Read the model definition and answer for the solid it produces. Units are mm, in the model's axes. A direction names the side the tool comes from. Coordinates: 2 decimals unless noted, no trailing zeros. Loops run counter-clockwise (first coordinate to the right, second up) from the corner with the lowest first, then second, coordinate; pieces in that order, holes last. Notation, with made-up numbers: (-36, 12) - (4, 12) arc R15 cw to (4, 22) - close; hole circle Ø9 at (78, 36.5). An arc over 180 degrees is marked (long way). Use one line per item in the form item = value.
from build123d import *

# Parameters (mm, degrees)
SKETCH1_W                    = 50.8
SKETCH1_H                    = 38.1
BOSS_EXTRUDE1_DEPTH          = 15.875
F_1_4_20_TAPPED_HOLE1_D      = 5.1054
CUT_EXTRUDE1_DEPTH           = 36.497579143
CUT_EXTRUDE1_DEPTH_BACK      = 36.497579143
SKETCH5_W                    = 73.284203365
SKETCH5_H                    = 114.763304797
CUT_EXTRUDE3_DEPTH           = 36.497579143
CUT_EXTRUDE3_DRAFT           = 45
CUT_EXTRUDE3_PROFILE_2_DEPTH = 36.497579143
CUT_EXTRUDE3_PROFILE_2_DRAFT = 45
CUT_EXTRUDE5_DEPTH           = 34.299680929
CUT_EXTRUDE5_DEPTH_BACK      = 34.299680929
SKETCH7_W                    = 138.535058429
SKETCH7_H                    = 124.054324336
SKETCH7_W_2                  = 31.75
SKETCH7_H_2                  = 70.377244636
F_1_4_20_TAPPED_HOLE2_D      = 5.1054
F_8_32_TAPPED_HOLE1_D        = 3.4544
F_8_32_TAPPED_HOLE1_DEPTH    = 12.7
F_8_32_TAPPED_HOLE1_TIP      = 1.037806461
CUT_EXTRUDE6_DEPTH           = 6.35
SKETCH14_R                   = 4.7625
CUT_EXTRUDE7_DEPTH           = 6.35


# Read off the part's stored shape, not the designer's step: LPattern1
with BuildPart() as part:
    # Sketch1 → Boss-Extrude1 (new body)
    with BuildSketch(Plane.XY):
        Rectangle(SKETCH1_W, SKETCH1_H)
    extrude(amount=BOSS_EXTRUDE1_DEPTH)

    # 1/4-20 Tapped Hole1 (through all)
    with Locations(Plane.XY.offset(15.875)):
        with Locations((7.6327, 12.7), (-7.6327, 12.7)):
            Hole(F_1_4_20_TAPPED_HOLE1_D / 2)

    # Sketch4 → Cut-Extrude1 (cut, two sides: drawn at the far end of the back side and taken through both)
    with BuildSketch(Plane.XY.offset(15.875).offset(-CUT_EXTRUDE1_DEPTH_BACK)):
        with BuildLine():
            Line((-39.282326984, 8.793789894), (-52.704404265, 33.364356416))
            Line((-52.704404265, 33.364356416), (0, 61.927684543))
            Line((0, 61.927684543), (62.667848215, 36.771765562))
            Line((62.667848215, 36.771765562), (48.5918884, 2.86093959))
            ThreePointArc((48.5918884, 2.86093959), (5.519661368, 18.637515941), (-39.282326984, 8.793789894))
        make_face()
    extrude(amount=CUT_EXTRUDE1_DEPTH + CUT_EXTRUDE1_DEPTH_BACK, mode=Mode.SUBTRACT)


with BuildPart() as cut_extrude3_tool:
    # Sketch5 → Cut-Extrude3 (with draft: the straight prism first)
    with BuildSketch(Plane.XY):
        with Locations((-42.992101682, 7.874882724)):
            Rectangle(SKETCH5_W, SKETCH5_H)
    extrude(amount=CUT_EXTRUDE3_DEPTH)
    # Cut-Extrude3: the draft: its side faces are tilted about the plane it starts from
    cut_extrude3_sides = [cut_extrude3_tool.faces().sort_by_distance(p)[0] for p in [
        (-42.992101682, 65.256535122, 18.248789571),
        (-79.634203365, 7.874882724, 18.248789571),
        (-42.992101682, -49.506769675, 18.248789571),
        (-6.35, 7.874882724, 18.248789571),
    ]]
    draft(cut_extrude3_sides, Plane.XY, CUT_EXTRUDE3_DRAFT)


with BuildPart() as part_1:
    add(part.part)

    # Cut-Extrude3: cut by cut_extrude3_tool
    add(cut_extrude3_tool.part, mode=Mode.SUBTRACT)


with BuildPart() as cut_extrude3_profile_2_tool:
    # Sketch5 → Cut-Extrude3 profile 2 (with draft: the straight prism first)
    with BuildSketch(Plane.XY):
        with Locations((42.992101682, 7.874882724)):
            Rectangle(SKETCH5_W, SKETCH5_H)
    extrude(amount=CUT_EXTRUDE3_PROFILE_2_DEPTH)
    # Cut-Extrude3 profile 2: the draft: its side faces are tilted about the plane it starts from
    cut_extrude3_profile_2_sides = [cut_extrude3_profile_2_tool.faces().sort_by_distance(p)[0] for p in [
        (42.992101682, 65.256535122, 18.248789571),
        (6.35, 7.874882724, 18.248789571),
        (42.992101682, -49.506769675, 18.248789571),
        (79.634203365, 7.874882724, 18.248789571),
    ]]
    draft(cut_extrude3_profile_2_sides, Plane.XY, CUT_EXTRUDE3_PROFILE_2_DRAFT)


with BuildPart() as part_2:
    add(part_1.part)

    # Cut-Extrude3 profile 2: cut by cut_extrude3_profile_2_tool
    add(cut_extrude3_profile_2_tool.part, mode=Mode.SUBTRACT)

    # Cut-Extrude4 cone 1 section (through the dimple's axis) → Cut-Extrude4 (revolve, cut)
    with BuildSketch(Plane(origin=(-7.6327, 12.7, 15.875), x_dir=(0, -1, 0), z_dir=(1, 0, 0))):
        Polygon((0, 0), (4.9276, 0), (0, 4.9276), align=None)
    revolve(axis=Axis((-7.6327, 12.7, 15.875), (0, 0, -1)), mode=Mode.SUBTRACT)

    # Cut-Extrude4 cone 2 section (through the dimple's axis) → Cut-Extrude4 cone 2 (revolve, cut)
    with BuildSketch(Plane(origin=(7.6327, 12.7, 15.875), x_dir=(0, -1, 0), z_dir=(1, 0, 0))):
        Polygon((0, 0), (4.9276, 0), (0, 4.9276), align=None)
    revolve(axis=Axis((7.6327, 12.7, 15.875), (0, 0, -1)), mode=Mode.SUBTRACT)

    # Sketch7 → Cut-Extrude5 (cut, two sides: drawn at the far end of the back side and taken through both)
    with BuildSketch(Plane.XY.offset(15.875).offset(-CUT_EXTRUDE5_DEPTH_BACK)):
        with Locations((-4.796027088, -12.18557991)):
            Rectangle(SKETCH7_W, SKETCH7_H)
        Rectangle(SKETCH7_W_2, SKETCH7_H_2, mode=Mode.SUBTRACT)
    extrude(amount=CUT_EXTRUDE5_DEPTH + CUT_EXTRUDE5_DEPTH_BACK, mode=Mode.SUBTRACT)

    # 1/4-20 Tapped Hole2 (through all)
    with Locations(Plane.XY.offset(15.875)):
        with Locations((0, -12.7), (0, 0)):
            Hole(F_1_4_20_TAPPED_HOLE2_D / 2)

    # #8-32 Tapped Hole1
    with Locations(Plane(origin=(0, 19.05, 0), x_dir=(-1, 0, 0), z_dir=(0, 1, 0))):
        with Locations((4.365625, 4.7625), (-4.365625, 4.7625)):
            Hole(F_8_32_TAPPED_HOLE1_D / 2, depth=F_8_32_TAPPED_HOLE1_DEPTH)
            with Locations((0, 0, -(F_8_32_TAPPED_HOLE1_DEPTH + F_8_32_TAPPED_HOLE1_TIP / 2))):  # 118° drill point
                Cone(0, F_8_32_TAPPED_HOLE1_D / 2, F_8_32_TAPPED_HOLE1_TIP, mode=Mode.SUBTRACT)

    # Sketch13 → Cut-Extrude6 (cut)
    with BuildSketch(Plane(origin=(0, 19.05, 0), x_dir=(-1, 0, 0), z_dir=(0, -1, 0))):
        with BuildLine():
            add(Edge.make_bspline(
                [(1.630169721, -12.065), (1.630169721, -8.8011), (-1.633730278, -8.8011), (-1.633730278, -12.065), (-1.633730278, -15.3289), (1.630169721, -15.3289), (1.630169721, -12.065)],
                knots=[0, 0, 0, 0, 0.5, 0.5, 0.5, 1, 1, 1, 1], degree=3, weights=[1, 0.333333333, 0.333333333, 1, 0.333333333, 0.333333333, 1]))
        make_face()
    extrude(amount=CUT_EXTRUDE6_DEPTH, mode=Mode.SUBTRACT)

    # LPattern1 outline → LPattern1 (revolve, cut)
    with BuildSketch(Plane(origin=(-7.6327, -6.35, 0), x_dir=(1, 0, 0), z_dir=(0, -1, 0))):
        Polygon((0, 0), (2.5527, 0), (2.5527, 13.5001), (4.9276, 15.875), (0, 15.875), align=None)
    revolve(axis=Axis((-7.6327, -6.35, 0), (0, 0, 1)), mode=Mode.SUBTRACT)

    # LPattern1 2 outline → LPattern1 2 (revolve, cut)
    with BuildSketch(Plane(origin=(7.6327, -6.35, 0), x_dir=(1, 0, 0), z_dir=(0, -1, 0))):
        Polygon((0, 0), (2.5527, 0), (2.5527, 13.5001), (4.9276, 15.875), (0, 15.875), align=None)
    revolve(axis=Axis((7.6327, -6.35, 0), (0, 0, 1)), mode=Mode.SUBTRACT)

    # Sketch14 → Cut-Extrude7 (cut)
    with BuildSketch(Plane.XY.offset(15.875)):
        Circle(SKETCH14_R)
        with Locations((0, -12.7)):
            Circle(SKETCH14_R)
    extrude(amount=-CUT_EXTRUDE7_DEPTH, mode=Mode.SUBTRACT)


solid = part_2.part
Item 1: Find the intervals of material crossed by L1, parallel to Y at x = 0, z = 7.75; L2, parallel to Y at x = -2.5, z = 14; L3, parallel to X at y = 12.7, z = 9.5, in increasing order.
Results below:
L1 = -19.05 to -15.25, -10.15 to -2.55, 2.55 to 18.82
L2 = -19.05 to -16.75, -8.65 to -4.05, 4.05 to 18.79
L3 = -15.85 to -10.19, -5.08 to 5.08, 10.19 to 15.85
Item 2: Each of these flat-tipped pins is pushed along its axis until it touches: P1, Ø1, axis at x = -0.5, z = 12, coming from the +Y side; P2, Ø6, axis at x = 0, y = -12.7, coming from the +Z side (3 decimals); P3, Ø6, axis at x = -7.63, y = 12.7, coming from the +Z side. Where does it stop, or does it pass through?
Results below:
P1 = 12.7
P2 = 9.525
P3 = 13.95
Item 3: Which of the six approach directions +Z, -Z, +X, -X, +Y, -Y give full straight-line access (tool end or side, diameter ignored) to faces 4 (the cylindrical face through (2.64, 12.48, 4.84)), 5 (the flat face through (2, -15, 9.525)), 6 (the flat face through (-15.875, -1, 13))?
Results below:
face_4 = +Y
face_5 = +Z
face_6 = +Z, -Z, -X, +Y, -Y
Item 4: The part is cut by section C-C on z = 9. Give the vertices of the cut face in (x, y).
Results below:
outline = (-15.35, -19.05) - (15.35, -19.05) - (15.35, 17.37) arc R81.94 ccw to (-15.35, 17.37) - close; hole circle Ø5.11 at (-7.63, -6.35); hole circle Ø5.11 at (-7.63, 12.7); hole circle Ø5.11 at (0, -12.7); hole circle Ø5.11 at (0, 0); hole circle Ø5.11 at (7.63, -6.35); hole circle Ø5.11 at (7.63, 12.7)
Item 5: For a pull along Z with two mould halves and no side action, classify faces 1 (the flat face through (2, -2, 9.525)), 2 (the cylindrical face through (-2.718, 12.479, 5.281)), 3 (the flat face through (-11.05, -0.5, 4.7)) as +Z half, -Z half, draft (parallel to the pull), parting line (faces both ways), or undercut.
Results below:
face_1 = +Z half
face_2 = undercut
face_3 = -Z half
Item 6: The part is cut by section B-B on y = 7. Count the separate pieces of the cut face and the enclosed holes in it, plus the area to 3 significant figures.
Results below:
separate_pieces = 1
enclosed_holes = 2
area = 395 mm²
